For this review, take the finished solid that the model builds, in its own axes (mm). A direction names the side the tool comes from. Round coordinates to 2 decimals unless told otherwise and drop trailing zeros. Order: outer loops, then holes, each group sorted by start corner. A loop starts at its lowest first (then second) coordinate and runs counter-clockwise, first axis right, second up. Notation, with made-up numbers: (17.25, 55) -> (65.25, 55) arc R18 cw to (65.25, 63) -> close; hole circle Ø6 at (56.25, -34.75). An arc over 180 degrees is marked (long way). Use a Markdown table: item, result. Add a question column.
1) Draft analysis for pull direction Y (two halves, no side actions). For faces 1 (the face through (0, 8.41, 12)), 2 (the face through (19, 0, 10)), 3 (the face through (0, 0, 0)), state which applies: pulls with the +Y half, pulls with the -Y half, needs draft (parallel to the pull), parting line crosses it, or undercut.
2) Clearance check with flat-ended pins moving along their axes: P1, Ø1.9, axis at x = -12, z = 18, coming from the -Y side; P2, Ø0.7, axis at x = 19, y = 0.5, coming from the -Z side. State where each tip first meets the part, or that it passes through.
3) Wall thickness on line 1 along X through (y, z) = (-1.75, 18); line 2 along X through (y, z) = (-0.5, 17); line 3 along X through (y, z) = (0.75, 9.75): over which ranges is each line inside the solid? List them lowest first. Write a range as [from, to].
4) Consider section C-C (y = 0). State the section outline as (x, z) points.
5) Machinability: for faces 4 (the face through (-11.446, 0.118, 19.065)), 5 (the face through (-17.49, -0.46, 4.93)), which of the approach directions +Z, -Z, +X, -X, +Y, -Y give a long, thin tool a straight path to every point of the face, cutting with its end or side? Answer none if there is none.
6) Consider section B-B (z = 9.25). State the section outline as (x, y) points.
7) Consider section D-D (z = 18.5). State the section outline as (x, y) points, plus the area to 3 significant figures.
8) Consider section A-A (x = 12). State the section outline as (y, z) points.
```python
from build123d import *

# Parameters (mm, degrees)
CROQUIS1_W              = 52.8
CROQUIS1_H              = 16.82
SALIENTE_EXTRUIR1_DEPTH = 30
CROQUIS2_R              = 1.2
CORTAR_EXTRUIR1_DEPTH   = 20
CROQUIS3_R              = 1.2
CORTAR_EXTRUIR2_DEPTH   = 10
CROQUIS4_W              = 52.8
CROQUIS4_H              = 16.82
CORTAR_EXTRUIR3_DEPTH   = 6


with BuildPart() as part:
    # Croquis1 → Saliente-Extruir1 (new body)
    with BuildSketch(Plane.XY):
        Rectangle(CROQUIS1_W, CROQUIS1_H)
    extrude(amount=SALIENTE_EXTRUIR1_DEPTH)

    # Croquis2 → Cortar-Extruir1 (cut)
    with BuildSketch(Plane(origin=(0, 8.41, 0), x_dir=(1, 0, 0), z_dir=(0, 1, 0))):
        with Locations((-12, -18)):
            Circle(CROQUIS2_R)
        with Locations((12, -18)):
            Circle(CROQUIS2_R)
    extrude(amount=-CORTAR_EXTRUIR1_DEPTH, mode=Mode.SUBTRACT)

    # Croquis3 → Cortar-Extruir2 (cut)
    with BuildSketch(Plane.XY):
        with Locations((18.6, 0)):
            Circle(CROQUIS3_R)
        with Locations((7, 0)):
            Circle(CROQUIS3_R)
        with Locations((-7, 0)):
            Circle(CROQUIS3_R)
        with Locations((-18.6, 0)):
            Circle(CROQUIS3_R)
    extrude(amount=CORTAR_EXTRUIR2_DEPTH, mode=Mode.SUBTRACT)

    # Croquis4 → Cortar-Extruir3 (cut)
    with BuildSketch(Plane.XY.offset(30)):
        Rectangle(CROQUIS4_W, CROQUIS4_H)
    extrude(amount=-CORTAR_EXTRUIR3_DEPTH, mode=Mode.SUBTRACT)


solid = part.part
```
Results list:
| question | item | result |
|---|---|---|
| 1 | face 1 | pulls with the +Y half |
| 1 | face 2 | undercut |
| 1 | face 3 | needs draft |
| 2 | P1 | through |
| 2 | P2 | z = 10 |
| 3 | line 1 | [-26.4, -13.2], [-10.8, 10.8], [13.2, 26.4] |
| 3 | line 2 | [-26.4, -12.66], [-11.34, 11.34], [12.66, 26.4] |
| 3 | line 3 | [-26.4, -19.54], [-17.66, -7.94], [-6.06, 6.06], [7.94, 17.66], [19.54, 26.4] |
| 4 | outline | (-26.4, 0) -> (-19.8, 0) -> (-19.8, 10) -> (-17.4, 10) -> (-17.4, 0) -> (-8.2, 0) -> (-8.2, 10) -> (-5.8, 10) -> (-5.8, 0) -> (5.8, 0) -> (5.8, 10) -> (8.2, 10) -> (8.2, 0) -> (17.4, 0) -> (17.4, 10) -> (19.8, 10) -> (19.8, 0) -> (26.4, 0) -> (26.4, 24) -> (-26.4, 24) -> close; hole circle Ø2.4 at (-12, 18); hole circle Ø2.4 at (12, 18) |
| 5 | face 4 | +Y, -Y |
| 5 | face 5 | -Z |
| 6 | outline | (-26.4, -8.41) -> (26.4, -8.41) -> (26.4, 8.41) -> (-26.4, 8.41) -> close; hole circle Ø2.4 at (-18.6, 0); hole circle Ø2.4 at (-7, 0); hole circle Ø2.4 at (7, 0); hole circle Ø2.4 at (18.6, 0) |
| 7 | outline | (-26.4, -8.41) -> (-13.09, -8.41) -> (-13.09, 8.41) -> (-26.4, 8.41) -> close; (-10.91, -8.41) -> (10.91, -8.41) -> (10.91, 8.41) -> (-10.91, 8.41) -> close; (13.09, -8.41) -> (26.4, -8.41) -> (26.4, 8.41) -> (13.09, 8.41) -> close |
| 7 | area | 815 mm2 |
| 8 | outline | (-8.41, 0) -> (8.41, 0) -> (8.41, 16.8) -> (-8.41, 16.8) -> close; (-8.41, 19.2) -> (8.41, 19.2) -> (8.41, 24) -> (-8.41, 24) -> close |
